Source: CAD feature listing. Evaluate the final solid. Frame: model axes, mm. Face numbers are marked on the shaded views. Coordinates: 2 decimals unless noted, no trailing zeros. Order: outer loops, then holes, each group sorted by start corner. A loop starts at its lowest first (then second) coordinate and runs counter-clockwise, first axis right, second up. Notation, with made-up numbers: (-7.5, -35) -> (7.5, -35) arc R14 cw to (7.5, -9) -> close; hole circle Ø11 at (22.5, 74.5). An arc over 180 degrees is marked (long way). Put each result on its own line as item: value.
from build123d import *

# Parameters (mm, degrees)
F0_W     = 70.5344155431
F0_H     = 70.8036422729
F0_R     = 1.8180060759
F1_DEPTH = 1.5
F2_DEPTH = 8
F4_D     = 5
F4_DEPTH = 10
F4_TIP   = 1.5021515476


# Not quite as in the source:
# - a feature names something its author has since deleted; it is built from what else it names


with BuildPart() as f1:
    # F0 (on Top) → F1 (new body)
    with BuildSketch(Plane.XY):
        Rectangle(F0_W, F0_H)
        with Locations((31.6813939209, -31.9532230342)):
            Circle(F0_R, mode=Mode.SUBTRACT)
        Polygon((-27.9887095094, 33.4018211365), (33.2672077715, 33.4018211365), (33.2672077715, -28.2499678433), (27.7495980263, -28.2499678433), (27.7495980263, -33.4018211365), (-33.2672077715, -33.4018211365), (-33.2672077715, 28.315147385), (-27.9887095094, 28.315147385), align=None, mode=Mode.SUBTRACT)
        with BuildLine():
            ThreePointArc((-30.620154253, 33.4018211365), (-29.8333233875, 32.6929228695), (-29.5415057982, 31.6748452405))
            ThreePointArc((-29.5415057982, 31.6748452405), (-33.093320688, 30.6567676116), (-30.620154253, 33.4018211365))
        make_face(mode=Mode.SUBTRACT)
        Polygon((33.2672077715, -28.2499678433), (33.2672077715, 33.4018211365), (-27.9887095094, 33.4018211365), (-27.9887095094, 28.315147385), (-33.2672077715, 28.315147385), (-33.2672077715, -33.4018211365), (27.7495980263, -33.4018211365), (27.7495980263, -28.2499678433), align=None)
        with BuildLine():
            ThreePointArc((-30.620154253, 33.4018211365), (-33.093320688, 30.6567676116), (-29.5415057982, 31.6748452405))
            ThreePointArc((-29.5415057982, 31.6748452405), (-29.8333233875, 32.6929228695), (-30.620154253, 33.4018211365))
        make_face()
        with Locations((31.6813939209, -31.9532230342)):
            Circle(F0_R)
    extrude(amount=F1_DEPTH)

    # F0 (on Top) → F2 (join)
    with BuildSketch(Plane.XY):
        Rectangle(F0_W, F0_H)
        with Locations((31.6813939209, -31.9532230342)):
            Circle(F0_R, mode=Mode.SUBTRACT)
        Polygon((-27.9887095094, 33.4018211365), (33.2672077715, 33.4018211365), (33.2672077715, -28.2499678433), (27.7495980263, -28.2499678433), (27.7495980263, -33.4018211365), (-33.2672077715, -33.4018211365), (-33.2672077715, 28.315147385), (-27.9887095094, 28.315147385), align=None, mode=Mode.SUBTRACT)
        with BuildLine():
            ThreePointArc((-30.620154253, 33.4018211365), (-29.8333233875, 32.6929228695), (-29.5415057982, 31.6748452405))
            ThreePointArc((-29.5415057982, 31.6748452405), (-33.093320688, 30.6567676116), (-30.620154253, 33.4018211365))
        make_face(mode=Mode.SUBTRACT)
    extrude(amount=F2_DEPTH)

    # F4
    with Locations(Plane(origin=(-35.2672077715, 0, 0), x_dir=(0, -1, 0), z_dir=(-1, 0, 0))):
        with Locations((0, 8)):
            Hole(F4_D / 2, depth=F4_DEPTH)
            with Locations((0, 0, -(F4_DEPTH + F4_TIP / 2))):  # 118° drill point
                Cone(0, F4_D / 2, F4_TIP, mode=Mode.SUBTRACT)


solid = f1.part
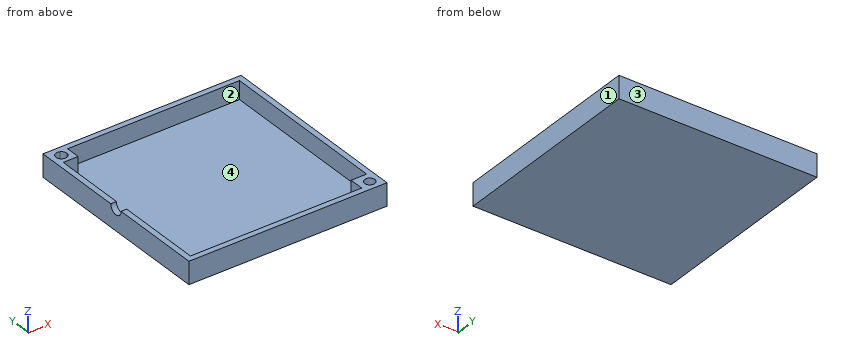
1. Ray query, line 1 along X through (y, z) = (-22, 6.5); line 2 along Y through (x, z) = (10.5, 4.75); line 3 along X through (y, z) = (30, 2.75). Return the intervals inside material, ascending.
Numbers:
line 1: x = -35.27 to -33.27, 33.27 to 35.27
line 2: y = -35.4 to -33.4, 33.4 to 35.4
line 3: x = -35.27 to -32.41, -30.52 to -27.99, 33.27 to 35.27
2. Cut plane B-B on x = 16. Output: boundary loops of the cut face in (y, z), plus the area to 3 significant figures.
Numbers:
outline: (-35.4, 0) -> (35.4, 0) -> (35.4, 8) -> (33.4, 8) -> (33.4, 1.5) -> (-33.4, 1.5) -> (-33.4, 8) -> (-35.4, 8) -> close
area: 132 mm2
3. First-contact query: pin 1 (2 mm diameter, centred on y = -0.5, z = 7, fed in from -X); pin 2 (5 mm diameter, centred on x = 22, y = 16, fed in from +Z). Flat tips, straight axial feed; report the tip coordinate or a pass-through.
Numbers:
pin 1: stops at x = 33.27
pin 2: stops at z = 1.5
4. Pull-direction query (X, two-part tool) for the marked faces 1, 2, 3 and 4; classes: pulls with the +X half, pulls with the -X half, needs draft (parallel to the pull), parting line crosses it, or undercut.
Numbers:
face 1: pulls with the +X half
face 2: undercut
face 3: needs draft
face 4: undercut
5. Cut plane A-A on y = -20. Output: boundary loops of the cut face in (x, z), plus the area to 3 significant figures.
Numbers:
outline: (-35.27, 0) -> (35.27, 0) -> (35.27, 8) -> (33.27, 8) -> (33.27, 1.5) -> (-33.27, 1.5) -> (-33.27, 8) -> (-35.27, 8) -> close
area: 132 mm2
6. Cut plane C-C on z = 6.5. Output: boundary loops of the cut face in (x, y).
Numbers:
outline: (-35.27, -35.4) -> (35.27, -35.4) -> (35.27, 35.4) -> (-35.27, 35.4) -> (-35.27, 2) -> (-33.27, 2) -> (-33.27, 28.32) -> (-27.99, 28.32) -> (-27.99, 33.4) -> (33.27, 33.4) -> (33.27, -28.25) -> (27.75, -28.25) -> (27.75, -33.4) -> (-33.27, -33.4) -> (-33.27, -2) -> (-35.27, -2) -> close; hole circle Ø3.84 at (-31.46, 31.67); hole circle Ø3.64 at (31.68, -31.95)
